Design review of the part built by this model. Coordinates are the model's own, in mm. Face numbers are marked on the shaded views. A direction names the side the tool comes from. Give positions to 0.01 mm unless a question says otherwise; leave off trailing zeros. Write each loop counter-clockwise with the first axis right and the second up, starting at its lowest first coordinate (ties: lowest second). Pieces come first, ordered by that corner, then holes. Notation, with made-up numbers: M -15.5,-25.5 L 33.5,-25.5 A28 cw 33.5,-3.5 Z; hole C -29,77 d4. An arc over 180 degrees is marked long. Answer in a Markdown table with one row per item.
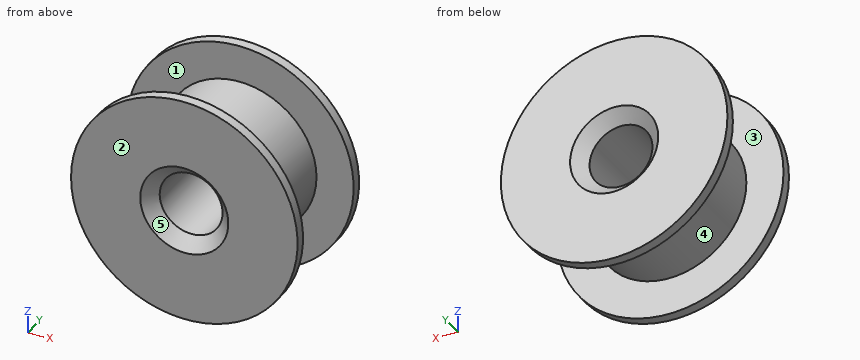
```python
from build123d import *

# Parameters (mm, degrees)
CHAMFER_1_SIZE = 1
CHAMFER_2_SIZE = 1


with BuildPart() as part:
    # Эскиз1 → Повернуть1 (revolve)
    with BuildSketch(Plane.XY):
        Polygon((-2.5, 0), (-9, 0), (-9, 0.8), (-6.05, 0.8), (-6.05, 8.2), (-9, 8.2), (-9, 9), (-2.5, 9), align=None)
    revolve(axis=Axis((0, 9, 0), (0, -1, 0)))

    # Фаска1
    chamfer_1_edges = [part.edges().sort_by_distance(p)[0] for p in [
        (2.5, 9, 0),
    ]]
    chamfer(chamfer_1_edges, length=CHAMFER_1_SIZE)

    # Фаска2
    chamfer_2_edges = [part.edges().sort_by_distance(p)[0] for p in [
        (2.5, 0, 0),
    ]]
    chamfer(chamfer_2_edges, length=CHAMFER_2_SIZE)


solid = part.part
```
1) The part is to be moulded in two halves that separate along Z. For the marked faces 3, 4 and 5, say which applies: released by +Z, released by -Z, zero draft, split by the parting line, or undercut.
Geometry says:
| item | result |
|---|---|
| face 3 | zero draft |
| face 4 | split by the parting line |
| face 5 | undercut |
2) Add section C-C (y = 2.75). Write out the cut boundary in (x, z), and give its area (3 significant figures).
Geometry says:
| item | result |
|---|---|
| outline | C 0,0 d12.1; hole C 0,0 d5 |
| area | 95.4 mm^2 |
3) For the marked faces 1 and 2, list the 3-axis set-ups (+Z, -Z, +X, -X, +Y, -Y) from which the entire face can be reached by the end or side of a thin tool; tool diameter is ignored.
Geometry says:
| item | result |
|---|---|
| face 1 | none |
| face 2 | +Z, -Z, +X, -X, -Y |
4) Insertion check: P1, Ø3, axis at y = 2.5, z = 2, coming from the -X side; P2, Ø2, axis at y = 3, z = -5.5, coming from the +X side; P3, Ø1, axis at y = 5.5, z = 4.5, coming from the +X side. Each pin has a flat end and moves straight along its axis. Give the tip position at first contact, or say it passes through.
Geometry says:
| item | result |
|---|---|
| P1 | x = -6.03 |
| P2 | x = 4.04 |
| P3 | x = 4.54 |
5) Add section B-B (z = 0). Write out the cut boundary in (x, y).
Geometry says:
| item | result |
|---|---|
| outline | M -9,0 L -3.5,0 L -2.5,1 L -2.5,8 L -3.5,9 L -9,9 L -9,8.2 L -6.05,8.2 L -6.05,0.8 L -9,0.8 Z; M 2.5,1 L 3.5,0 L 9,0 L 9,0.8 L 6.05,0.8 L 6.05,8.2 L 9,8.2 L 9,9 L 3.5,9 L 2.5,8 Z |
6) Add section A-A (x = 0). Write out the cut boundary in (y, z), and give its area (3 significant figures).
Geometry says:
| item | result |
|---|---|
| outline | M 0,-9 L 0.8,-9 L 0.8,-6.05 L 8.2,-6.05 L 8.2,-9 L 9,-9 L 9,-3.5 L 8,-2.5 L 1,-2.5 L 0,-3.5 Z; M 0,3.5 L 1,2.5 L 8,2.5 L 9,3.5 L 9,9 L 8.2,9 L 8.2,6.05 L 0.8,6.05 L 0.8,9 L 0,9 Z |
| area | 71.3 mm^2 |
7) Add section D-D (z = 5). Write out the cut boundary in (x, y), and give its area (3 significant figures).
Geometry says:
| item | result |
|---|---|
| outline | M -7.48,0 L 7.48,0 L 7.48,0.8 L 3.41,0.8 L 3.41,8.2 L 7.48,8.2 L 7.48,9 L -7.48,9 L -7.48,8.2 L -3.41,8.2 L -3.41,0.8 L -7.48,0.8 Z |
| area | 74.4 mm^2 |
8) To check wall thickness, follow probe 1 along X at (y, z) = (2.75, 0); probe 2 along Y at (x, z) = (-2, -6). State the ranges of each line that lie inside material, in increasing order. Write a range as [from, to].
Geometry says:
| item | result |
|---|---|
| probe 1 | [-6.05, -2.5], [2.5, 6.05] |
| probe 2 | [0, 0.8], [8.2, 9] |
